Autodesk Inventor part; units mm, degrees
ref_plane "YZ Plane" through (0, 0, 0) normal (1, 0, 0) x (0, 1, 0)
ref_plane "XZ Plane" through (0, 0, 0) normal (0, 1, 0) x (-1, 0, 0)
ref_plane "XY Plane" through (0, 0, 0) normal (0, 0, 1) x (1, 0, 0)
sketch "Sketch1" plane through (0, 0, 0) normal (0, 1, 0) x (-1, 0, 0)
  line L0 (27.775, -33.32) -> (-27.775, -33.32)
  line L1 (-27.775, -33.32) -> (-27.775, 33.32)
  line L2 (-27.775, 33.32) -> (27.775, 33.32)
  line L3 (27.775, 33.32) -> (27.775, -33.32)
  line L4 (27.775, -33.32) -> (-27.775, 33.32) construction
  line L5 (-27.775, -33.32) -> (27.775, 33.32) construction
  line L6 (26.775, -32.3) -> (-26.775, -32.3)
  line L7 (-26.775, -32.3) -> (-26.775, 32.3)
  line L8 (-26.775, 32.3) -> (26.775, 32.3)
  line L9 (26.775, 32.3) -> (26.775, -32.3)
  line L10 (26.775, -32.3) -> (-26.775, 32.3) construction
  line L11 (-26.775, -32.3) -> (26.775, 32.3) construction
  point P0 (0, 0)
  dimension "d0" = 66.64
  dimension "d1" = 55.55
  dimension "d2" = 64.6
  dimension "d3" = 53.55
extrude "Extrusion1" add sketch "Sketch1" along normal blind 1 contours L0 L1 L2 L3 | L6 L7 L8 L9
sketch "Sketch2" plane through (0, 1, 0) normal (0, 1, 0) x (1, 0, 0)
  line L0 (-26.775, 32.15) -> (26.775, 32.15)
  line L1 (26.775, 32.15) -> (26.775, -32.15)
  line L2 (26.775, -32.15) -> (-26.775, -32.15)
  line L3 (-26.775, -32.15) -> (-26.775, 32.15)
  line L4 (-26.775, 32.15) -> (26.775, -32.15) construction
  line L5 (26.775, 32.15) -> (-26.775, -32.15) construction
  line L6 (-26.775, 32.15) -> (-24.775, 32.15)
  line L7 (-24.775, 32.15) -> (-24.775, 30.15)
  line L8 (-24.775, 30.15) -> (-26.775, 30.15) construction
  line L9 (-26.775, 30.15) -> (-26.775, 32.15)
  line L10 (-24.775, 30.15) -> (-19.775, 30.15)
  line L11 (-19.775, 30.15) -> (-19.775, 32.15)
  line L12 (-19.775, 32.15) -> (-24.775, 32.15)
  line L13 (-24.775, 32.15) -> (-24.775, 30.15)
  line L14 (26.775, 32.15) -> (24.775, 32.15)
  line L15 (24.775, 32.15) -> (24.775, 30.15)
  line L16 (24.775, 30.15) -> (26.775, 30.15) construction
  line L17 (26.775, 30.15) -> (26.775, 32.15)
  line L18 (24.775, 32.15) -> (19.775, 32.15)
  line L19 (19.775, 32.15) -> (19.775, 30.15)
  line L20 (19.775, 30.15) -> (24.775, 30.15)
  line L21 (24.775, 30.15) -> (24.775, 32.15)
  line L22 (-26.775, -32.15) -> (-24.775, -32.15)
  line L23 (-24.775, -32.15) -> (-24.775, -30.15)
  line L24 (-24.775, -30.15) -> (-26.775, -30.15) construction
  line L25 (-26.775, -30.15) -> (-26.775, -32.15)
  line L26 (-24.775, -30.15) -> (-19.775, -30.15)
  line L27 (-19.775, -30.15) -> (-19.775, -32.15)
  line L28 (-19.775, -32.15) -> (-24.775, -32.15)
  line L29 (-24.775, -32.15) -> (-24.775, -30.15)
  line L30 (26.775, -32.15) -> (24.775, -32.15)
  line L31 (24.775, -32.15) -> (24.775, -30.45)
  line L32 (24.775, -30.45) -> (26.775, -30.45) construction
  line L33 (26.775, -30.45) -> (26.775, -32.15)
  line L34 (24.775, -30.45) -> (19.775, -30.45)
  line L35 (19.775, -30.45) -> (19.775, -32.15)
  line L36 (19.775, -32.15) -> (24.775, -32.15)
  line L37 (24.775, -32.15) -> (24.775, -30.45)
  point P0 (0, 0)
  point P1 (-24.775, -32.15)
  point P2 (-24.775, 32.15)
  dimension "d6" = 53.55
  dimension "d7" = 64.3
  dimension "d8" = 2
  dimension "d9" = 2
  dimension "d10" = 5
  dimension "d11" = 2
  dimension "d12" = 2
  dimension "d13" = 5
  dimension "d14" = 2
  dimension "d15" = 2
  dimension "d16" = 5
  dimension "d17" = 2
  dimension "d18" = 5
extrude "Extrusion2" add sketch "Sketch2" along normal blind 2 contours L0 L11 L10 L7 | L0 L15 L20 L19 | L23 L26 L27 L2 | L35 L34 L31 L2
sketch "Sketch3" plane through (0, 1, 0) normal (0, 1, 0) x (1, 0, 0)
  line L0 (27.775, 33.32) -> (-27.775, 33.32)
  line L1 (0, 33.32) -> (0, -4.68)
  line L2 (0, -4.68) -> (5, -4.68)
  line L3 (0, -4.68) -> (-5, -4.68)
  line L4 (-5, -4.68) -> (-5, -6.68)
  line L5 (-5, -6.68) -> (5, -6.68)
  line L6 (5, -6.68) -> (5, -4.68)
  point P0 (0, 0)
  dimension "d21" = 38
  dimension "d22" = 5
  dimension "d23" = 5
  dimension "d24" = 2
extrude "Extrusion3" add sketch "Sketch3" along normal blind 4
properties part number "bottomplate"
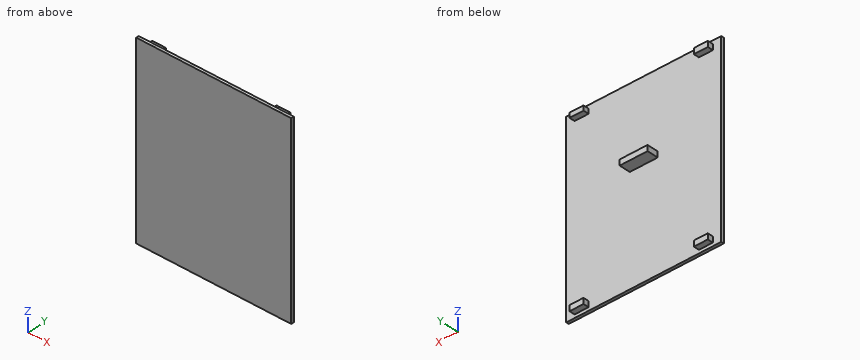
The listing builds one solid part. Answer for the finished solid, in the listing's coordinates (mm). Give positions to 0.01 mm unless a question says otherwise; leave off trailing zeros. Loops run counter-clockwise (first coordinate to the right, second up) from the corner with the lowest first, then second, coordinate; pieces in that order, holes last. Notation, with made-up numbers: M -31.5,14.25 L -8.5,14.25 A16 cw -8.5,25.25 Z; hole C -23,31.25 d4. An arc over 180 degrees is marked long. One line per item, written item: value.
Q1. Flat-ended cylindrical pins translate along their axes: P1, Ø0.6, axis at y = 2, z = -31, coming from the -X side (3 decimals); P2, Ø2, axis at x = -23, y = 2.5, coming from the -Z side; P3, Ø2, axis at y = 3, z = 5.5, coming from the +X side. Find the tip coordinate at first contact, or state that the pin passes through.
Working result:
P1: stops at x = -24.775
P2: stops at z = -32.15
P3: stops at x = 5
Q2. A cutting plane is placed at B-B on z = -1. Determine the outline of the cut face in (x, y) (3 decimals), then the cut area to 4 significant figures.
Working result:
outline: M -27.775,0 L 27.775,0 L 27.775,1 L -27.775,1 Z
area: 55.55 mm^2
Q3. A cutting plane is placed at C-C on x = -1.5. Determine the outline of the cut face in (y, z).
Working result:
outline: M 0,-33.32 L 1,-33.32 L 1,4.68 L 5,4.68 L 5,6.68 L 1,6.68 L 1,33.32 L 0,33.32 Z
Q4. A cutting plane is placed at D-D on x = -19. Determine the outline of the cut face in (y, z).
Working result:
outline: M 0,-33.32 L 1,-33.32 L 1,33.32 L 0,33.32 Z
Q5. A cutting plane is placed at A-A on x = 21. Determine the outline of the cut face in (y, z), then the cut area to 3 significant figures.
Working result:
outline: M 0,-33.32 L 1,-33.32 L 1,-32.15 L 3,-32.15 L 3,-30.15 L 1,-30.15 L 1,30.45 L 3,30.45 L 3,32.15 L 1,32.15 L 1,33.32 L 0,33.32 Z
area: 74.0 mm^2
Q6. Find the intervals of material crossed by line 1 (Z direction, x = 22, y = 1.05); line 2 (Y direction, x = -19, z = 2.5); line 3 (Z direction, x = -0.5, y = 2.05), in increasing order. Write a range as from..to.
Working result:
line 1: z = -32.15..-30.15, 30.45..32.15
line 2: y = 0..1
line 3: z = 4.68..6.68
